Geometry: final body of the model. Coordinates: model frame, mm. Face numbers are marked on the shaded views. A direction names the side the tool comes from. Round coordinates to 2 decimals unless told otherwise and drop trailing zeros. Order: outer loops, then holes, each group sorted by start corner. A loop starts at its lowest first (then second) coordinate and runs counter-clockwise, first axis right, second up. Notation, with made-up numbers: (80.5, 83) -> (136.5, 83) arc R31 ccw to (136.5, 114) -> close; hole circle Ø1 at (71.5, 76). An arc over 180 degrees is marked (long way). Put each result on its own line as item: value.
```python
from build123d import *

# Parameters (mm, degrees)
SKETCH1_W           = 100
SKETCH1_H           = 50
BOSS_EXTRUDE1_DEPTH = 40
SKETCH2_W           = 90
SKETCH2_H           = 40
CUT_EXTRUDE1_DEPTH  = 30
SKETCH3_W           = 36
SKETCH3_H           = 12
BOSS_EXTRUDE2_DEPTH = 30
FILLET1_R           = 2
DRAFT2_ANGLE        = 10
DRAFT5_ANGLE        = -8
SKETCH4_R           = 8
CUT_EXTRUDE2_DEPTH  = 27
CUT_EXTRUDE2_TAPER  = 3


with BuildPart() as part:
    # Sketch1 → Boss-Extrude1 (new body)
    with BuildSketch(Plane(origin=(0, 0, 0), x_dir=(1, 0, 0), z_dir=(0, 1, 0))):
        Rectangle(SKETCH1_W, SKETCH1_H)
    extrude(amount=BOSS_EXTRUDE1_DEPTH)

    # Sketch2 → Cut-Extrude1 (cut)
    with BuildSketch(Plane(origin=(0, 40, 0), x_dir=(1, 0, 0), z_dir=(0, 1, 0))):
        Rectangle(SKETCH2_W, SKETCH2_H)
    extrude(amount=-CUT_EXTRUDE1_DEPTH, mode=Mode.SUBTRACT)

    # Sketch3 → Boss-Extrude2 (add)
    with BuildSketch(Plane(origin=(50, 0, 0), x_dir=(0, 0, -1), z_dir=(1, 0, 0))):
        with Locations((0, 20)):
            Rectangle(SKETCH3_W, SKETCH3_H)
    extrude(amount=BOSS_EXTRUDE2_DEPTH)

    # Fillet1
    fillet1_edges = [part.edges().sort_by_distance(p)[0] for p in [
        (50, 26, 0),
        (50, 14, 0),
        (80, 26, 0),
        (80, 14, 0),
    ]]
    fillet(fillet1_edges, radius=FILLET1_R)

    # Draft2
    draft2_faces = [part.faces().sort_by_distance(p)[0] for p in [
        (0, 20, -25),
        (0, 20, 25),
    ]]
    draft(draft2_faces, Plane(origin=(0, 0, 0), x_dir=(0, 0, -1), z_dir=(0, -1, 0)), DRAFT2_ANGLE)

    # Draft5
    draft5_faces = [part.faces().sort_by_distance(p)[0] for p in [
        (0, 25, 20),
        (0, 25, -20),
    ]]
    draft(draft5_faces, Plane.ZX.offset(40), DRAFT5_ANGLE)

    # Sketch4 → Cut-Extrude2 (cut, through all)
    with BuildSketch(Plane(origin=(0, 26, 0), x_dir=(1, 0, 0), z_dir=(0, 1, 0))):
        with Locations((65, 0)):
            Circle(SKETCH4_R)
    extrude(amount=-CUT_EXTRUDE2_DEPTH, taper=CUT_EXTRUDE2_TAPER, mode=Mode.SUBTRACT)


solid = part.part
```
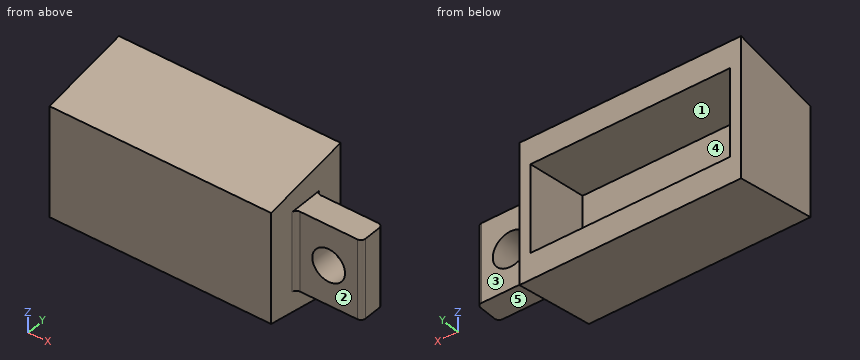
1. Cut plane D-D on y = 37. Return loops of the section in (x, z), and give its area (3 significant figures).
Ans:
outline: (-50, -31.52) -> (50, -31.52) -> (50, 31.52) -> (-50, 31.52) -> close; hole (-45, -20.42) -> (45, -20.42) -> (45, 20.42) -> (-45, 20.42) -> close
area: 2,630 mm²
2. Contact query for flat-ended pins moving along their axis: P1, Ø13, axis at x = 66, y = 23, coming from the +Z side; P2, Ø15, axis at y = 26.5, z = -4.5, coming from the +X side; P3, Ø21, axis at x = 70.5, z = -5.5, coming from the +Y side; P4, Ø5, axis at x = 0, z = -4, coming from the +Y side. Output: stop coordinate, or through.
Ans:
P1: z = 18
P2: x = 80
P3: y = 26
P4: y = 10
3. Material intervals for probe 1 along X at (y, z) = (22.5, -20); probe 2 along X at (y, z) = (24.5, 6.5); probe 3 along X at (y, z) = (21, -12.5), sorted ascending.
Ans:
probe 1: -50 to -45, 45 to 50
probe 2: -50 to -45, 45 to 60.47, 69.53 to 79.94
probe 3: -50 to -45, 45 to 80
4. Cut plane C-C on x = -13.5. Return loops of the section in (y, z), and give its area (3 significant figures).
Ans:
outline: (0, -25) -> (40, -32.05) -> (40, -20) -> (10, -24.22) -> (10, 24.22) -> (40, 20) -> (40, 32.05) -> (0, 25) -> close
area: 956 mm²
5. Draft query along Z for the marked faces 3, 4 and 5. Return one class per face: +Z half, -Z half, draft (parallel to the pull), parting line (faces both ways), or undercut.
Ans:
face 3: draft
face 4: undercut
face 5: -Z half
6. Set-up query: the marked faces 1 and 2. Return all of +Z, -Z, +X, -X, +Y, -Y with unobstructed straight access to the full face (end or side cutting, diameter ignored); none if empty.
Ans:
face 1: none
face 2: +Z, -Z, +X, -Y
7. Cut plane B-B on y = 30.5. Return loops of the section in (x, z).
Ans:
outline: (-50, -30.38) -> (50, -30.38) -> (50, 30.38) -> (-50, 30.38) -> close; hole (-45, -21.34) -> (45, -21.34) -> (45, 21.34) -> (-45, 21.34) -> close
8. Cut plane A-A on x = 65. Return loops of the section in (y, z), and give its area (3 significant figures).
Ans:
outline: (14, -18) -> (26, -18) -> (26, -8) -> (14, -7.37) -> close; (14, 7.37) -> (26, 8) -> (26, 18) -> (14, 18) -> close
area: 248 mm²
